```python
from build123d import *

# Parameters (mm, degrees)
SKETCH_1_R           = 10.2
EXTRUDE_1_DEPTH      = 25.1
SKETCH_2_OUTSIDE_W   = 30.048
SKETCH_2_OUTSIDE_H   = 30.048
SKETCH_2_OUTSIDE_W_2 = 29.995014986
SKETCH_2_OUTSIDE_H_2 = 15.4
CUT_EXTRUDE_1_DEPTH  = 54.1
SKETCH_3_R           = 3.15
EXTRUDE_2_DEPTH      = 2.1
FILLET_1_R           = 0.5
SKETCH_4_R           = 3.075
EXTRUDE_3_DEPTH      = 1.7
SKETCH_6_R           = 1
EXTRUDE_4_DEPTH      = 9.8
SKETCH_7_R           = 1.1
CUT_EXTRUDE_2_DEPTH  = 3


with BuildPart() as part:
    # 草图1 → 凸台-拉伸1 (new body)
    with BuildSketch(Plane(origin=(0, 0, 0), x_dir=(0, 0, -1), z_dir=(1, 0, 0))):
        Circle(SKETCH_1_R)
    extrude(amount=EXTRUDE_1_DEPTH)

    # 草图2 outside → 切除-拉伸1 (cut)
    with BuildSketch(Plane.ZY):
        Rectangle(SKETCH_2_OUTSIDE_W, SKETCH_2_OUTSIDE_H)
        Rectangle(SKETCH_2_OUTSIDE_W_2, SKETCH_2_OUTSIDE_H_2, mode=Mode.SUBTRACT)
    extrude(amount=-CUT_EXTRUDE_1_DEPTH, mode=Mode.SUBTRACT)

    # 草图3 → 凸台-拉伸2 (add)
    with BuildSketch(Plane(origin=(25.1, 0, 0), x_dir=(0, 0, -1), z_dir=(1, 0, 0))):
        Circle(SKETCH_3_R)
    extrude(amount=EXTRUDE_2_DEPTH)

    # 圆角1
    fillet_1_edges = [part.edges().sort_by_distance(p)[0] for p in [
        (27.2, 0, 3.15),
    ]]
    fillet(fillet_1_edges, radius=FILLET_1_R)

    # 草图4 → 凸台-拉伸3 (add)
    with BuildSketch(Plane.ZY):
        Circle(SKETCH_4_R)
    extrude(amount=EXTRUDE_3_DEPTH)

    # 草图6 → 凸台-拉伸4 (add)
    with BuildSketch(Plane.ZY):
        Circle(SKETCH_6_R)
    extrude(amount=EXTRUDE_4_DEPTH)

    # 草图7 → 切除-拉伸2 (cut)
    with BuildSketch(Plane.ZY):
        with Locations((6.2, 0)):
            Circle(SKETCH_7_R)
        with Locations((-6.2, 0)):
            Circle(SKETCH_7_R)
    extrude(amount=-CUT_EXTRUDE_2_DEPTH, mode=Mode.SUBTRACT)


solid = part.part
```
Can you work these out from the model? Positions are in its coordinate system, mm. A direction names the side the tool comes from. Round coordinates to 2 decimals unless told otherwise and drop trailing zeros. Loops run counter-clockwise (first coordinate to the right, second up) from the corner with the lowest first, then second, coordinate; pieces in that order, holes last. Notation, with made-up numbers: M 75,24 L 92,24 A31 ccw 92,56 Z; hole C 77,79 d7. An arc over 180 degrees is marked long. Write item = value, one per line. Start each with the question number.
(1) Suppose I cut it at C-C on z = 6.2. Write out the boundary of the cut face in (x, y).
(2) Suppose I cut it at D-D on y = -4. Write out the boundary of the cut face in (x, z), plus the area to 3 significant figures.
(3) Suppose I cut it at A-A on z = 0. Write out the boundary of the cut face in (x, y) (3 decimals), plus the area to 3 significant figures.
(4) I'm going to push flat-ended pins straight in: P1, Ø7, axis at y = -1, z = -1.5, coming from the -X side; P2, Ø3, axis at y = 0, z = -6.2, coming from the -X side; P3, Ø5, axis at y = 5.5, z = -7.5, coming from the +X side. Where does each tip first touch, or does it pass through?
(5) I need wall thicknesses on line 1 along Y through (x, z) = (1.3, 6.2); line 2 along X through (y, z) = (-3, 6.75); line 3 along X through (y, z) = (1, -6). Which ranges of each line are inside material? Lowest first, please.
(6) If we mould it in two halves opening along Y, with no side actions, what happens to faces 1 (the face through (0, -3.3, 0.1)), 2 (the face through (1.5, 0, -7.3)), 3 (the face through (12.4, 0.1, 10.2)), 4 (the face through (1.5, 0, 5.1))? For each: released by +Y, released by -Y, zero draft, split by the parting line, or undercut.
(7) Which directions (+Z, -Z, +X, -X, +Y, -Y) give clear straight access to the entire face, cutting with the end or side of a thin tool? Please do faces 5 (the face through (25.889, -1.917, 2.5)), 6 (the face through (-6, -1, 0)), 7 (the face through (12, -7.7, 0)).
(8) Suppose I cut it at B-B on x = 8. Write out the boundary of the cut face in (y, z).
Answer block:
q1.outline = M 0,-7.7 L 25.1,-7.7 L 25.1,7.7 L 0,7.7 L 0,1.1 L 3,1.1 L 3,-1.1 L 0,-1.1 Z
q2.outline = M 0,-9.38 L 25.1,-9.38 L 25.1,9.38 L 0,9.38 Z
q2.area = 471 mm²
q3.outline = M -9.8,-1 L -1.7,-1 L -1.7,-3.075 L 0,-3.075 L 0,-7.7 L 25.1,-7.7 L 25.1,-3.15 L 26.7,-3.15 A0.5 ccw 27.2,-2.65 L 27.2,2.65 A0.5 ccw 26.7,3.15 L 25.1,3.15 L 25.1,7.7 L 0,7.7 L 0,3.075 L -1.7,3.075 L -1.7,1 L -9.8,1 Z
q3.area = 426 mm²
q4.P1 = -9.8
q4.P2 = 0
q4.P3 = 25.1
q5.line_1 = -7.7 to -1.1, 1.1 to 7.7
q5.line_2 = 0 to 25.1
q5.line_3 = 3 to 25.1
q6.face_1 = zero draft
q6.face_2 = undercut
q6.face_3 = split by the parting line
q6.face_4 = undercut
q7.face_5 = +X
q7.face_6 = -X
q7.face_7 = +Z, -Z, +X, -X, -Y
q8.outline = M -7.7,-6.69 A10.2 ccw 7.7,-6.69 L 7.7,6.69 A10.2 ccw -7.7,6.69 Z
